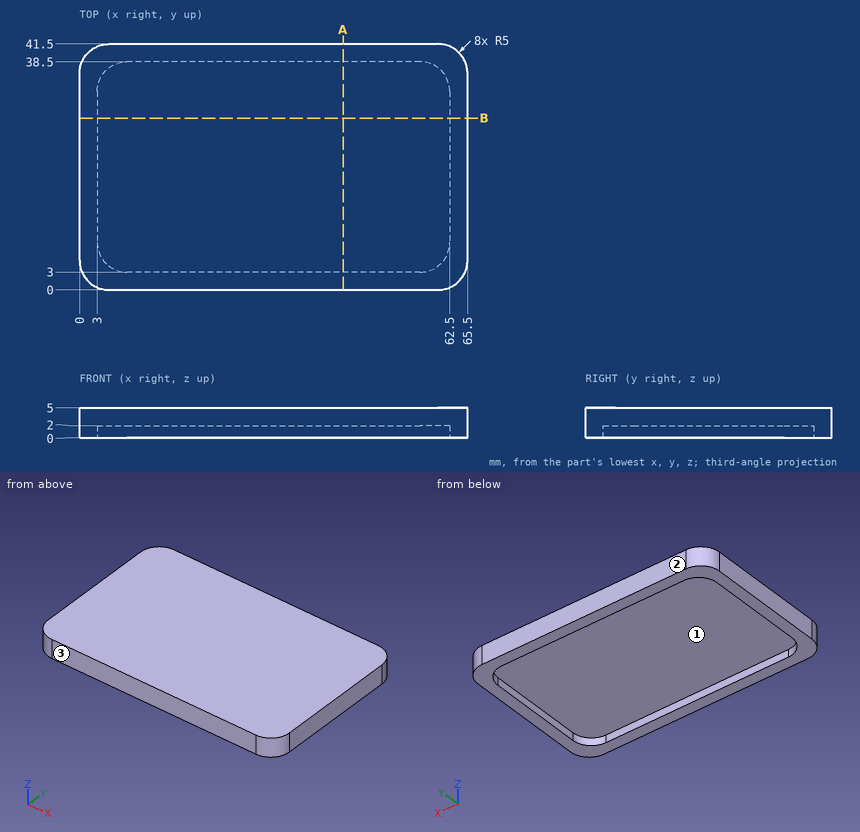
The figure shows three views and two pictorial views of one solid part (mm, origin at its lowest corner). Answer the questions. Give positions to 0.01 mm unless a question says otherwise; leave off trailing zeros. Write each loop counter-clockwise with the first axis right and the second up, starting at its lowest first coordinate (ties: lowest second). Pieces come first, ordered by that corner, then holes. Notation, with made-up numbers: (34.5, 45.5) - (54.5, 45.5) arc R10 ccw to (54.5, 53.5) - close; hole circle Ø10 at (2.25, -18.5). An arc over 180 degrees is marked (long way). Return JSON: item names as keys, results as strings.
Q1. For a pull along Y with two mould halves and no side action, classify the marked faces 1, 2 and 3 as released by +Y, released by -Y, zero draft, split by the parting line, or undercut.
Reply:
{"face 1": "undercut", "face 2": "released by +Y", "face 3": "released by -Y"}
Q2. Consider line 1 along Y through (x, z) = (24.5, 0.4); line 2 along X through (y, z) = (14.5, 1.85); line 3 along Z through (x, y) = (43.5, 35). Determine where each line is inside the solid, lowest interval first. Write a range as [from, to].
Reply:
{"line 1": "[0, 3], [38.5, 41.5]", "line 2": "[0, 3], [62.5, 65.5]", "line 3": "[2, 5]"}
Q3. A cutting plane is placed at B-B, the plane y = 29. Determine the outline of the cut face in (x, z), and give its area (4 significant figures).
Reply:
{"outline": "(0, 0) - (3, 0) - (3, 2) - (62.5, 2) - (62.5, 0) - (65.5, 0) - (65.5, 5) - (0, 5) - close", "area": "208.5 mm²"}
Q4. A cutting plane is placed at A-A, the plane x = 44.5. Determine the outline of the cut face in (y, z).
Reply:
{"outline": "(0, 0) - (3, 0) - (3, 2) - (38.5, 2) - (38.5, 0) - (41.5, 0) - (41.5, 5) - (0, 5) - close"}
Q5. Given P1, Ø0.6, axis at y = 14.5, z = 1, coming from the -X side; P2, Ø18, axis at x = 45.5, y = 13, coming from the -Z side, each flat-ended and moving along its own axis, determine where each tip first touches the part or whether it passes through.
Reply:
{"P1": "x = 0", "P2": "z = 2"}
